Could you check a few things on this model? Use its own coordinates, in mm. Face numbers are marked on the shaded views. Coordinates: 2 decimals unless noted, no trailing zeros. Order: outer loops, then holes, each group sorted by start corner. A loop starts at its lowest first (then second) coordinate and runs counter-clockwise, first axis right, second up. Notation, with made-up numbers: (-33, -4.5) - (-27, -4.5) arc R19 cw to (-27, 22.5) - close; hole circle Ø3 at (2, 68). An arc over 180 degrees is marked (long way). One line per item, written item: value.
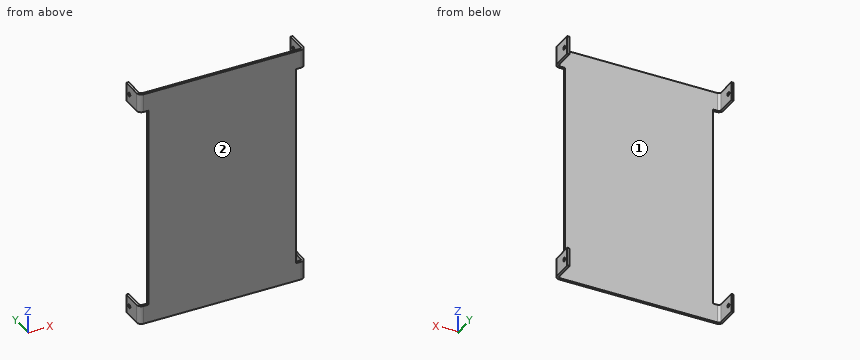
from build123d import *

# Parameters (mm, degrees)
BASE_FLANGE1_DEPTH      = 330.2
SKETCH21_R              = 2.5796875
CUT_EXTRUDE1_DEPTH      = 403.964415799
CUT_EXTRUDE2_DEPTH      = 403.716679596
CUT_EXTRUDE2_DEPTH_BACK = 403.716679596
SKETCH22_W              = 50.8
SKETCH22_H              = 279.4


# Sheet-metal steps are written as plain solids
with BuildPart() as part:
    # Sketch7 → Base-Flange1 (new body)
    with BuildSketch(Plane.XY):
        with BuildLine():
            Line((-228.6, 33.02), (-228.6, 6.35))
            ThreePointArc((-228.6, 6.35), (-226.740128061, 1.859871939), (-222.25, 0))
            Line((-222.25, 0), (-6.35, 0))
            ThreePointArc((-6.35, 0), (-1.859871939, 1.859871939), (0, 6.35))
            Line((0, 6.35), (0, 33.02))
            Line((0, 33.02), (-3.175, 33.02))
            Line((-3.175, 33.02), (-3.175, 6.35))
            ThreePointArc((-3.175, 6.35), (-4.10493597, 4.10493597), (-6.35, 3.175))
            Line((-6.35, 3.175), (-222.25, 3.175))
            ThreePointArc((-222.25, 3.175), (-224.49506403, 4.10493597), (-225.425, 6.35))
            Line((-225.425, 6.35), (-225.425, 33.02))
            Line((-225.425, 33.02), (-228.6, 33.02))
        make_face()
    extrude(amount=BASE_FLANGE1_DEPTH)

    # Sketch21 → Cut-Extrude1 (cut, through all)
    with BuildSketch(Plane.ZY.offset(228.6)):
        with Locations((12.7, 25.4)):
            Circle(SKETCH21_R)
        with Locations((317.5, 25.4)):
            Circle(SKETCH21_R)
    extrude(amount=-CUT_EXTRUDE1_DEPTH, mode=Mode.SUBTRACT)

    # Sketch22 → Cut-Extrude2 (cut, two sides: drawn at the far end of the back side and taken through both)
    with BuildSketch(Plane(origin=(0, 3.175, 0), x_dir=(1, 0, 0), z_dir=(0, 1, 0)).offset(-CUT_EXTRUDE2_DEPTH_BACK)):
        with Locations((-241.3, -165.1)):
            Rectangle(SKETCH22_W, SKETCH22_H)
        with Locations((12.7, -165.1)):
            Rectangle(SKETCH22_W, SKETCH22_H)
    extrude(amount=CUT_EXTRUDE2_DEPTH + CUT_EXTRUDE2_DEPTH_BACK, mode=Mode.SUBTRACT)


solid = part.part
Item 1: I'm going to push flat-ended pins straight in: pin 1 Ø10 at (x, y) = (-222, 20.5) entering from -Z; pin 2 Ø5 at (x, z) = (-85.5, 159) entering from +Y (3 decimals); pin 3 Ø8 at (x, y) = (-101.5, 9) entering from +Z; pin 4 Ø3.5 at (y, z) = (1.5, 119.5) entering from +X. Where does each tip first touch, or does it pass through?
Conclusion:
pin 1: z = 0
pin 2: y = 3.175
pin 3: through
pin 4: x = -12.7
Item 2: I want a section at C-C on x = -149.5. Please give me the cut outline in (y, z) (3 decimals), then the cut area to 3 significant figures.
Conclusion:
outline: (0, 0) - (3.175, 0) - (3.175, 330.2) - (0, 330.2) - close
area: 1,050 mm²
Item 3: I want a section at B-B on z = 309. Please give me the cut outline in (x, y) (3 decimals), then the cut area to 3 significant figures.
Conclusion:
outline: (-228.6, 6.35) arc R6.35 ccw to (-222.25, 0) - (-6.35, 0) arc R6.35 ccw to (0, 6.35) - (0, 33.02) - (-3.175, 33.02) - (-3.175, 6.35) arc R3.175 cw to (-6.35, 3.175) - (-222.25, 3.175) arc R3.175 cw to (-225.425, 6.35) - (-225.425, 33.02) - (-228.6, 33.02) - close
area: 902 mm²
Item 4: I want a section at A-A on y = 13. Please give me the cut outline in (x, z) (3 decimals), then the cut area to 3 significant figures.
Conclusion:
outline: (-228.6, 0) - (-225.425, 0) - (-225.425, 25.4) - (-228.6, 25.4) - close; (-228.6, 304.8) - (-225.425, 304.8) - (-225.425, 330.2) - (-228.6, 330.2) - close; (-3.175, 0) - (0, 0) - (0, 25.4) - (-3.175, 25.4) - close; (-3.175, 304.8) - (0, 304.8) - (0, 330.2) - (-3.175, 330.2) - close
area: 323 mm²
Item 5: I want a section at D-D on z = 230.5. Please give me the cut outline in (x, y) (3 decimals).
Conclusion:
outline: (-215.9, 0) - (-12.7, 0) - (-12.7, 3.175) - (-215.9, 3.175) - close
Item 6: Thinking about a two-plate mould opening in Y: for the marked faces 1 and 2, which applies, pulls with the +Y half, pulls with the -Y half, needs draft (parallel to the pull), parting line crosses it, or undercut?
Conclusion:
face 1: pulls with the +Y half
face 2: pulls with the -Y half
Item 7: If I drill on probe 1 along Z at (x, y) = (-1, 25); probe 2 along Y at (x, z) = (-19.5, 282.5) (3 decimals); probe 3 along Y at (x, z) = (-1.7, 12.7), over which ranges is the centre line in solid material (lowest first)?
Conclusion:
probe 1: 0 to 10.15, 15.25 to 25.4, 304.8 to 314.95, 320.05 to 330.2
probe 2: 0 to 3.175
probe 3: 2.03 to 22.82, 27.98 to 33.02
